from build123d import *

# Parameters (mm, degrees)
F0_W           = 25.4
F0_H           = 25.4
F1_DEPTH       = 10.668
F2_R           = 2.54
F4_D           = 6.35
F4_CSINK_D     = 12.7
F4_CSINK_ANGLE = 90


with BuildPart() as f1:
    # F0 (on Top) → F1 (new body)
    with BuildSketch(Plane.XY):
        Rectangle(F0_W, F0_H)
    extrude(amount=F1_DEPTH)

    # F2
    f2_edges = [f1.edges().sort_by_distance(p)[0] for p in [
        (0, -12.7, 10.668),
        (0, 12.7, 10.668),
        (12.7, 0, 10.668),
        (-12.7, 0, 10.668),
    ]]
    fillet(f2_edges, radius=F2_R)

    # F4 (through all)
    with Locations(Plane.XY.offset(10.668)):
        with Locations((0, 0)):
            CounterSinkHole(F4_D / 2, F4_CSINK_D / 2, counter_sink_angle=F4_CSINK_ANGLE)


solid = f1.part
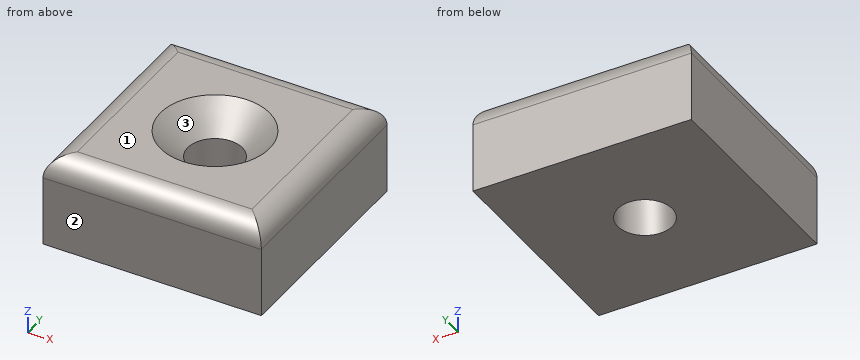
Could you check a few things on this model? Use its own coordinates, in mm. Face numbers are marked on the shaded views. Round coordinates to 2 decimals unless told otherwise and drop trailing zeros. Loops run counter-clockwise (first coordinate to the right, second up) from the corner with the lowest first, then second, coordinate; pieces in that order, holes last. Notation, with made-up numbers: (59.5, -1.75) - (86.5, -1.75) arc R22 cw to (86.5, 11.25) - close; hole circle Ø10 at (45.25, 17). An arc over 180 degrees is marked (long way). Write item = value, one per line.
1) I need wall thicknesses on line 1 along Y through (x, z) = (0, 4.5) (3 decimals); line 2 along Y through (x, z) = (1.75, 3.25). Which ranges of each line are inside material? Lowest first, please. Write a range as from..to.
Computed:
line_1 = -12.7..-3.175, 3.175..12.7
line_2 = -12.7..-2.65, 2.65..12.7
2) If we mould it in two halves opening along Y, with no side actions, what happens to the marked faces 1, 2 and 3? For each: pulls with the +Y half, pulls with the -Y half, needs draft (parallel to the pull), parting line crosses it, or undercut.
Computed:
face_1 = needs draft
face_2 = pulls with the -Y half
face_3 = undercut
3) Imagine slicing it at C-C (z = 6). Please give me the cut outline in (x, y) (3 decimals), and give its area (3 significant figures).
Computed:
outline = (-12.7, -12.7) - (12.7, -12.7) - (12.7, 12.7) - (-12.7, 12.7) - close; hole circle Ø6.35 at (0, 0)
area = 613 mm2
4) Imagine slicing it at D-D (z = 9). Please give me the cut outline in (x, y).
Computed:
outline = (-12.55, -12.55) - (12.55, -12.55) - (12.55, 12.55) - (-12.55, 12.55) - close; hole circle Ø9.36 at (0, 0)
5) Imagine slicing it at A-A (y = 0). Please give me the cut outline in (x, z) (3 decimals).
Computed:
outline = (-12.7, 0) - (-3.175, 0) - (-3.175, 7.493) - (-6.35, 10.668) - (-10.16, 10.668) arc R2.54 ccw to (-12.7, 8.128) - close; (3.175, 0) - (12.7, 0) - (12.7, 8.128) arc R2.54 ccw to (10.16, 10.668) - (6.35, 10.668) - (3.175, 7.493) - close
